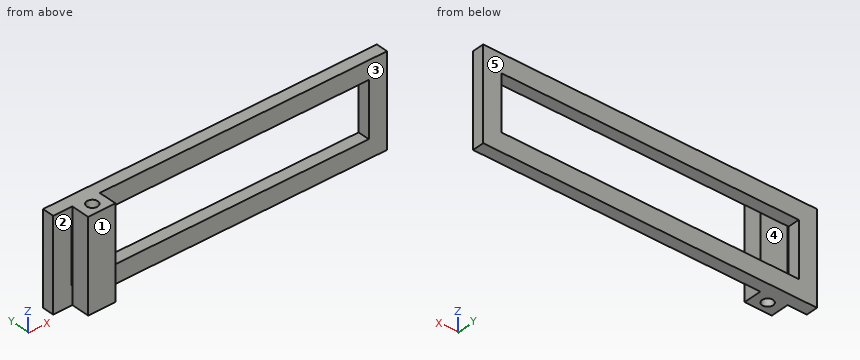
```python
from build123d import *

# Parameters (mm, degrees)
SKETCH_1_W          = 183
SKETCH_1_H          = 6.5
EXTRUDE_1_DEPTH     = 10
SKETCH_2_W          = 10
SKETCH_2_H          = 6.5
EXTRUDE_2_DEPTH     = 40
EXTRUDE_3_REACH     = 182.198
SKETCH_3_W          = 10
SKETCH_3_H          = 6.5
SKETCH_7_W          = 15
SKETCH_7_H          = 50
EXTRUDE_5_DEPTH     = 10
CUT_EXTRUDE_2_REACH = 191.971
SKETCH_8_R          = 3


with BuildPart() as part:
    # 草图1 → 凸台-拉伸1 (new body)
    with BuildSketch(Plane.XY):
        with Locations((91.5, 3.25)):
            Rectangle(SKETCH_1_W, SKETCH_1_H)
    extrude(amount=-EXTRUDE_1_DEPTH)

    # 草图2 → 凸台-拉伸2 (add)
    with BuildSketch(Plane(origin=(0, 0, -10), x_dir=(-1, 0, 0), z_dir=(0, 0, -1))):
        with Locations((-178, 3.25)):
            Rectangle(SKETCH_2_W, SKETCH_2_H)
        with Locations((-5, 3.25)):
            Rectangle(SKETCH_2_W, SKETCH_2_H)
    extrude(amount=EXTRUDE_2_DEPTH)

    # 草图3 → 凸台-拉伸3 (add, up to next)
    with BuildSketch(Plane(origin=(10, 0, 0), x_dir=(0, 0, -1), z_dir=(1, 0, 0)), mode=Mode.PRIVATE) as extrude_3_sk1:
        with Locations((45, 3.25)):
            Rectangle(SKETCH_3_W, SKETCH_3_H)
    extrude_3_tool1 = extrude(extrude_3_sk1.sketch, amount=EXTRUDE_3_REACH, mode=Mode.PRIVATE) - part.part
    add(extrude_3_tool1.solids().sort_by_distance((10, 3.25, -45))[0])

    # 草图7 → 凸台-拉伸5 (add)
    with BuildSketch(Plane.XZ):
        with Locations((18, -25)):
            Rectangle(SKETCH_7_W, SKETCH_7_H)
    extrude(amount=EXTRUDE_5_DEPTH)

    # 草图8 → 切除-拉伸2 (cut, up to next)
    with BuildSketch(Plane.XY, mode=Mode.PRIVATE) as cut_extrude_2_sk1:
        with Locations((18, -4)):
            Circle(SKETCH_8_R)
    cut_extrude_2_tool1 = extrude(cut_extrude_2_sk1.sketch, amount=-CUT_EXTRUDE_2_REACH, mode=Mode.PRIVATE) & part.part
    add(cut_extrude_2_tool1.solids().sort_by_distance((18, -4, 0))[0], mode=Mode.SUBTRACT)


solid = part.part
```
Model file for the job. Use its own axes, mm. Face numbers are marked on the shaded views. A direction names the side the tool comes from. Give positions to 0.01 mm unless a question says otherwise; leave off trailing zeros. Loops run counter-clockwise (first coordinate to the right, second up) from the corner with the lowest first, then second, coordinate; pieces in that order, holes last. Notation, with made-up numbers: (34, 6) - (70, 6) arc R29 cw to (70, 38) - close; hole circle Ø7 at (-35, -29). An arc over 180 degrees is marked (long way). One line per item, written item: value. Start each with the question number.
1. Probe L1, parallel to Z at x = 76.5, y = 0.25; L2, parallel to Y at x = 18, z = -39; L3, parallel to X at y = 1.75, z = -16.5. List the from-to ranges inside material, lowest first. Write a range as from..to.
2. Which spindle directions (+Z, -Z, +X, -X, +Y, -Y) get a long thin tool onto all of the face, cutting with end or side? Do the marked faces 1, 2 and 3. Say none if no direction does.
3. Pull direction Z, two halves, no side cores. Call the marked faces 4 and 5: pulls with the +Z half, pulls with the -Z half, needs draft (parallel to the pull), parting line crosses it, or undercut.
4. Pin check, flat tips, straight feed: pin 1 (5 mm diameter, centred on x = 5.5, z = -34.5, fed in from -Y); pin 2 (8 mm diameter, centred on x = 20.5, z = -29, fed in from +Y); pin 3 (1.5 mm diameter, centred on y = -4.5, z = -6.5, fed in from +X); pin 4 (1.5 mm diameter, centred on x = 119.5, y = -1.5, fed in from +Z). Stop position of each tip, or through.
5. Slice it at B-B (y = -4). List the corners of the cut face in (x, z), plus the area to 3 significant figures.
6. Slice it at A-A (x = 100). List the corners of the cut face in (y, z).
7. Slice it at C-C (z = -14.5). List the corners of the cut face in (x, y).
8. Slice it at D-D (y = 4.25). List the corners of the cut face in (x, z).
Solution:
1. L1: z = -50..-40, -10..0
1. L2: y = -10..-7, -1..0
1. L3: x = 0..10, 173..183
2. face 1: +Z, -Z, +X, -X, -Y
2. face 2: +Z, -Z, -X, -Y
2. face 3: +Z, -Z, +X, -Y
3. face 4: undercut
3. face 5: needs draft
4. pin 1: stops at y = 0
4. pin 2: stops at y = 0
4. pin 3: stops at x = 25.5
4. pin 4: passes through
5. outline: (10.5, -50) - (15, -50) - (15, 0) - (10.5, 0) - close; (21, -50) - (25.5, -50) - (25.5, 0) - (21, 0) - close
5. area: 450 mm^2
6. outline: (0, -50) - (6.5, -50) - (6.5, -40) - (0, -40) - close; (0, -10) - (6.5, -10) - (6.5, 0) - (0, 0) - close
7. outline: (0, 0) - (10, 0) - (10, 6.5) - (0, 6.5) - close; (10.5, -10) - (25.5, -10) - (25.5, 0) - (10.5, 0) - close; (173, 0) - (183, 0) - (183, 6.5) - (173, 6.5) - close; hole circle Ø6 at (18, -4)
8. outline: (0, -50) - (183, -50) - (183, 0) - (0, 0) - close; hole (10, -40) - (173, -40) - (173, -10) - (10, -10) - close
